```python
from build123d import *

# Parameters (mm, degrees)
F0_R     = 11
F1_DEPTH = 10
F2_W     = 1
F2_H     = 3.693367015
F3_DEPTH = 4


with BuildPart() as f1:
    # F0 (on Front) → F1 (new body)
    with BuildSketch(Plane.XZ):
        with BuildLine():
            Line((-3.0604514879, 9.8880870564), (-7.4054963655, 9.8880870564))
            ThreePointArc((-7.4054963655, 9.8880870564), (-35.3291650939, -3.9419436711), (-6.351978263, -15.4015976163))
            Line((-6.351978263, -15.4015976163), (-3.0604514879, -6.7412075195))
            Line((-3.0604514879, -6.7412075195), (-3.0604514879, 3.9817849485))
            Line((-3.0604514879, 3.9817849485), (-3.0604514879, 7.9859482356))
            Line((-3.0604514879, 7.9859482356), (-3.0604514879, 9.8880870564))
        make_face()
        with Locations((-18.2939400691, -3.2322899852)):
            Circle(F0_R, mode=Mode.SUBTRACT)
        Polygon((-1.0604514879, 9.8880870564), (-3.0604514879, 9.8880870564), (-3.0604514879, 7.9859482356), (-1.0604514879, 7.9859482356), (-1.0604514879, 7.0903341385), (0.2310752873, 7.0903341385), (0.2310752873, 10.7837011535), (-1.0604514879, 10.7837011535), align=None)
    extrude(amount=F1_DEPTH)

    # F2 (on face) → F3 (cut)
    with BuildSketch(Plane.YZ.offset(0.2310752873)):
        with Locations((-9.5, 8.937017646)):
            Rectangle(F2_W, F2_H)
        with Locations((-0.5, 8.937017646)):
            Rectangle(F2_W, F2_H)
    extrude(amount=-F3_DEPTH, mode=Mode.SUBTRACT)


solid = f1.part
```
For this review, take the finished solid that the model builds, in its own axes (mm). A direction names the side the tool comes from. Coordinates: 2 decimals unless noted, no trailing zeros. Write each loop counter-clockwise with the first axis right and the second up, starting at its lowest first coordinate (ties: lowest second). Pieces come first, ordered by that corner, then holes.
(1) For pin 1 Ø1.5 at (y, z) = (-2, 3.5) entering from -X; pin 2 Ø0.8 at (y, z) = (-0.5, 8.5) entering from +X; pin 3 Ø4 at (x, z) = (-1, 10) entering from -Y, all flat-tipped, find the tip position at first contact; note any pin that passes through.
(2) Add section D-D on x = -30.5. Give the boundary of the cut face in (y, z).
(3) Wall thickness on probe 1 along X at (y, z) = (-8.5, -3); probe 2 along Z at (x, y) = (-18, -9.5); probe 3 along Z at (x, y) = (-10.5, -3.25): over which ranges is each line inside the solid? List them lowest first.
(4) Add section B-B on z = 4.5. Give the boundary of the cut face in (x, y).
(5) Add section C-C on y = -7.75. Give the boundary of the cut face in (x, z).
(6) Tool access review of faces 1 (the face through (-1.06, -4.9, 7.5)), 2 (the face through (0, -5, 7.09)), 3 (the face through (-3.769, -9.5, 8.5)): name each direction out of +Z, -Z, +X, -X, +Y, -Y from which nothing blocks a thin tool from reaching the whole face with its end or side.
(7) The part is to be moulded in two halves that separate along X. For faces 4 (the face through (-1.06, -4.9, 10.3)), 5 (the face through (-7.8, -4.93, 0.07)), 6 (the face through (-27, -10, 5)), 7 (the face through (-3.769, -0.5, 8.5)), say which applies: +X half, -X half, draft (parallel to the pull), parting line (faces both ways), or undercut.
(8) Add section A-A on x = -12.5. Give the boundary of the cut face in (y, z).
Answer sheet:
1. pin 1: stops at x = -34.26
1. pin 2: stops at x = -3.77
1. pin 3: stops at y = -9
2. outline: (-10, -15.14) - (0, -15.14) - (0, 8.67) - (-10, 8.67) - close
3. probe 1: x = -35.34 to -29.29, -7.3 to -3.06
3. probe 2: z = -20.28 to -14.23, 7.76 to 13.82
3. probe 3: z = -18.4 to -10.99, 4.53 to 11.93
4. outline: (-33.49, -10) - (-26.12, -10) - (-26.12, 0) - (-33.49, 0) - close; (-10.47, -10) - (-3.06, -10) - (-3.06, 0) - (-10.47, 0) - close
5. outline: (-7.41, 9.89) arc R17.05 ccw (long way) to (-6.35, -15.4) - (-3.06, -6.74) - (-3.06, 7.99) - (-1.06, 7.99) - (-1.06, 7.09) - (0.23, 7.09) - (0.23, 10.78) - (-1.06, 10.78) - (-1.06, 9.89) - close; hole circle Ø22 at (-18.29, -3.23)
6. face 1: -Z, +Y, -Y
6. face 2: -Z, +X, +Y, -Y
6. face 3: +Z, +X, -Y
7. face 4: undercut
7. face 5: undercut
7. face 6: draft
7. face 7: +X half
8. outline: (-10, -19.27) - (0, -19.27) - (0, -12.58) - (-10, -12.58) - close; (-10, 6.12) - (0, 6.12) - (0, 12.8) - (-10, 12.8) - close
